from build123d import *

# Parameters (mm, degrees)
SKETCH1_W                    = 40
SKETCH1_H                    = 40
SKETCH1_R                    = 4.25
SKETCH1_R_2                  = 2.25
BOSS_EXTRUDE1_DEPTH          = 3
SKETCH3_R                    = 9.25
SKETCH3_R_2                  = 4.25
BOSS_EXTRUDE2_DEPTH          = 5
CUT_EXTRUDE_THIN1_DEPTH      = 29.722813233
CUT_EXTRUDE_THIN1_DEPTH_BACK = 3
SKETCH2_W                    = 3
SKETCH2_H                    = 20
CHAMFER1_SIZE                = 5
CHAMFER2_SIZE                = 2


with BuildPart() as part:
    # Sketch1 → Boss-Extrude1 (new body)
    with BuildSketch(Plane(origin=(0, 0, 0), x_dir=(1, 0, 0), z_dir=(0, 1, 0))):
        Rectangle(SKETCH1_W, SKETCH1_H)
        with Locations(Location((0, 0, 0), (0, 0, 270))):
            Circle(SKETCH1_R, mode=Mode.SUBTRACT)
        with Locations(Location((-12, -12, 0), (0, 0, 270))):
            Circle(SKETCH1_R_2, mode=Mode.SUBTRACT)
        with Locations(Location((-12, 12, 0), (0, 0, 270))):
            Circle(SKETCH1_R_2, mode=Mode.SUBTRACT)
        with Locations(Location((12, 12, 0), (0, 0, 270))):
            Circle(SKETCH1_R_2, mode=Mode.SUBTRACT)
        with Locations(Location((12, -12, 0), (0, 0, 270))):
            Circle(SKETCH1_R_2, mode=Mode.SUBTRACT)
    extrude(amount=BOSS_EXTRUDE1_DEPTH)

    # Sketch3 → Boss-Extrude2 (add)
    with BuildSketch(Plane(origin=(0, 3, 0), x_dir=(1, 0, 0), z_dir=(0, 1, 0))):
        with Locations(Location((0, 0, 0), (0, 0, 270))):
            Circle(SKETCH3_R)
        with Locations(Location((0, 0, 0), (0, 0, 270))):
            Circle(SKETCH3_R_2, mode=Mode.SUBTRACT)
    extrude(amount=BOSS_EXTRUDE2_DEPTH)

    # Sketch2 → Cut-Extrude-Thin1 (cut, two sides: drawn at the far end of the back side and taken through both)
    with BuildSketch(Plane(origin=(0, 3, 0), x_dir=(1, 0, 0), z_dir=(0, 1, 0)).offset(-CUT_EXTRUDE_THIN1_DEPTH_BACK)):
        with Locations((0, 10)):
            Rectangle(SKETCH2_W, SKETCH2_H)
    extrude(amount=CUT_EXTRUDE_THIN1_DEPTH + CUT_EXTRUDE_THIN1_DEPTH_BACK, mode=Mode.SUBTRACT)

    # Chamfer1
    chamfer1_edges = [part.edges().sort_by_distance(p)[0] for p in [
        (20, 1.5, 20),
        (-20, 1.5, 20),
        (-20, 1.5, -20),
        (20, 1.5, -20),
    ]]
    chamfer(chamfer1_edges, length=CHAMFER1_SIZE)

    # Chamfer2
    chamfer2_edges = [part.edges().sort_by_distance(p)[0] for p in [
        (0, 3, 9.25),
    ]]
    chamfer(chamfer2_edges, length=CHAMFER2_SIZE)


solid = part.part
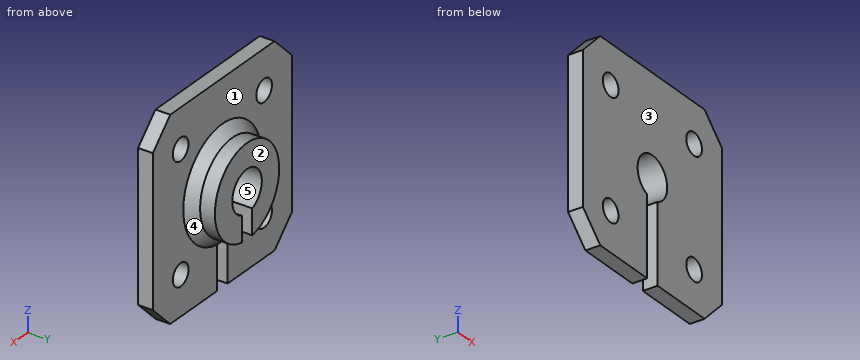
Design review of the part built by this model. Coordinates are the model's own, in mm. Face numbers are marked on the shaded views. A direction names the side the tool comes from. Coordinates: 2 decimals unless noted, no trailing zeros. Loops run counter-clockwise (first coordinate to the right, second up) from the corner with the lowest first, then second, coordinate; pieces in that order, holes last.
Item 1: Clearance check with a flat-ended pin moving along its axis: pin 1 (4 mm diameter, centred on x = 5.5, y = 6, fed in from -Z). State where the tip first meets the part, or that it passes through.
Completed:
pin 1: stops at z = -8.92
Item 2: Add section A-A (z = -12). Write out the cut boundary in (x, y).
Completed:
outline: (-20, 0) - (-14.25, 0) - (-14.25, 3) - (-20, 3) - close; (-9.75, 0) - (-1.5, 0) - (-1.5, 3) - (-9.75, 3) - close; (1.5, 0) - (9.75, 0) - (9.75, 3) - (1.5, 3) - close; (14.25, 0) - (20, 0) - (20, 3) - (14.25, 3) - close
Item 3: Add section D-D (x = 12). Write out the cut boundary in (y, z).
Completed:
outline: (0, -20) - (3, -20) - (3, -14.25) - (0, -14.25) - close; (0, -9.75) - (3, -9.75) - (3, 9.75) - (0, 9.75) - close; (0, 14.25) - (3, 14.25) - (3, 20) - (0, 20) - close
Item 4: For the marked faces 1 and 2, list the 3-axis set-ups (+Z, -Z, +X, -X, +Y, -Y) from which the entire face can be reached by the end or side of a thin tool; tool diameter is ignored.
Completed:
face 1: +Y
face 2: +Z, -Z, +X, -X, +Y
Item 5: Add section B-B (z = 0). Write out the cut boundary in (x, y).
Completed:
outline: (-20, 0) - (-4.25, 0) - (-4.25, 8) - (-9.25, 8) - (-9.25, 5) - (-11.25, 3) - (-20, 3) - close; (4.25, 0) - (20, 0) - (20, 3) - (11.25, 3) - (9.25, 5) - (9.25, 8) - (4.25, 8) - close
Item 6: Add section C-C (z = 12). Write out the cut boundary in (x, y).
Completed:
outline: (-20, 0) - (-14.25, 0) - (-14.25, 3) - (-20, 3) - close; (-9.75, 0) - (9.75, 0) - (9.75, 3) - (-9.75, 3) - close; (14.25, 0) - (20, 0) - (20, 3) - (14.25, 3) - close
Item 7: Draft analysis for pull direction Z (two halves, no side actions). For the marked faces 3, 4 and 5, state which applies: pulls with the +Z half, pulls with the -Z half, needs draft (parallel to the pull), parting line crosses it, or undercut.
Completed:
face 3: needs draft
face 4: parting line crosses it
face 5: undercut
Item 8: Wall thickness on L1, parallel to X at y = 1.2, z = 12; L2, parallel to X at y = 1.05, z = -12; L3, parallel to X at y = 2.25, z = -5.5: over which ranges is each line inside the solid? List them lowest first.
Completed:
L1: x = -20 to -14.25, -9.75 to 9.75, 14.25 to 20
L2: x = -20 to -14.25, -9.75 to -1.5, 1.5 to 9.75, 14.25 to 20
L3: x = -20 to -1.5, 1.5 to 20
